Geometry check sheet. Reference: the model listing, model coordinates, mm. A direction names the side the tool comes from. Round coordinates to 2 decimals unless told otherwise and drop trailing zeros. Write each loop counter-clockwise with the first axis right and the second up, starting at its lowest first coordinate (ties: lowest second). Pieces come first, ordered by that corner, then holes. Notation, with made-up numbers: (53, 78.25) - (78, 78.25) arc R30 cw to (78, 111.25) - close; hole circle Ø7 at (17, -32.5). An arc over 180 degrees is marked (long way). Return JSON: item names as keys, results as strings.
```python
from build123d import *

# Parameters (mm, degrees)
SKETCH_W        = 20
SKETCH_H        = 40
PAD_DEPTH       = 1.75
SKETCH001_W     = 7.5
SKETCH001_H     = 5.5
PAD001_DEPTH    = 3.5
POCKET_DEPTH    = 5.5
SKETCH003_W     = 4.5
SKETCH003_H     = 0.4
POCKET001_DEPTH = 5
SKETCH004_W     = 10
SKETCH004_H     = 7.25
PAD002_DEPTH    = 5
SKETCH005_W     = 8.4
SKETCH005_H     = 4
POCKET002_DEPTH = 5
SKETCH006_W     = 0.8
SKETCH006_H     = 0.8
PAD003_DEPTH    = 4.5
SKETCH007_W     = 6
SKETCH007_H     = 6
SKETCH007_W_2   = 4.5
SKETCH007_H_2   = 4.5
SKETCH007_W_3   = 0.75
SKETCH007_H_3   = 1.5
SKETCH007_W_4   = 2.9
SKETCH007_H_4   = 1.2
SKETCH007_W_5   = 1.5
SKETCH007_H_5   = 0.75
PAD004_DEPTH    = 0.5
SKETCH008_W     = 3
SKETCH008_H     = 4
PAD005_DEPTH    = 1
SKETCH009_R     = 0.8
PAD006_DEPTH    = 0.75
SKETCH010_W     = 6
SKETCH010_H     = 5
POCKET003_DEPTH = 0.5


with BuildPart() as part:
    # Sketch → Pad (new body)
    with BuildSketch(Plane.XY):
        Rectangle(SKETCH_W, SKETCH_H)
    extrude(amount=PAD_DEPTH)

    # Sketch001 (on Face6 of Pad) → Pad001 (join)
    with BuildSketch(Plane.XY.offset(1.75)):
        with Locations((0, -17.75)):
            Rectangle(SKETCH001_W, SKETCH001_H)
    extrude(amount=PAD001_DEPTH)

    # Sketch002 (on Face11 of Pad001) → Pocket (cut)
    with BuildSketch(Plane.XZ.offset(20.5)):
        Polygon((-3.75, 5.25), (-3.75, 4.5), (-3.25, 5.25), align=None)
        Polygon((-3.75, 1.75), (-3.75, 3.5), (-2.75, 1.75), align=None)
    pocket = extrude(amount=-POCKET_DEPTH, mode=Mode.SUBTRACT)

    # Mirrored: Pocket across YZ
    add(pocket.mirror(Plane.YZ), mode=Mode.SUBTRACT)

    # Sketch003 (on Face10 of Mirrored) → Pocket001 (cut)
    with BuildSketch(Plane.XZ.offset(20.5)):
        Polygon((-3.166667, 5), (-3.5, 4.5), (-3.5, 3.75), (-2.5, 2), (2.5, 2), (3.5, 3.75), (3.5, 4.5), (3.166667, 5), align=None)
        with Locations((0, 4.1)):
            Rectangle(SKETCH003_W, SKETCH003_H, mode=Mode.SUBTRACT)
    extrude(amount=-POCKET001_DEPTH, mode=Mode.SUBTRACT)

    # Sketch004 (on Face5 of Pocket001) → Pad002 (join)
    with BuildSketch(Plane.XY.offset(1.75)):
        with Locations((0, 16.875)):
            Rectangle(SKETCH004_W, SKETCH004_H)
    extrude(amount=PAD002_DEPTH)

    # Sketch005 (on Face15 of Pad002) → Pocket002 (cut)
    with BuildSketch(Plane(origin=(0, 20.5, 0), x_dir=(-1, 0, 0), z_dir=(0, 1, 0))):
        with Locations((0, 4.25)):
            Rectangle(SKETCH005_W, SKETCH005_H)
    extrude(amount=-POCKET002_DEPTH, mode=Mode.SUBTRACT)

    # Sketch006 (on Face35 of Pocket002) → Pad003 (join)
    with BuildSketch(Plane(origin=(0, 15.5, 0), x_dir=(-1, 0, 0), z_dir=(0, 1, 0))):
        with Locations((-2.76, 4.25)):
            Rectangle(SKETCH006_W, SKETCH006_H)
        with Locations((-0.92, 4.25)):
            Rectangle(SKETCH006_W, SKETCH006_H)
        with Locations((0.92, 4.25)):
            Rectangle(SKETCH006_W, SKETCH006_H)
        with Locations((2.76, 4.25)):
            Rectangle(SKETCH006_W, SKETCH006_H)
    extrude(amount=PAD003_DEPTH)

    # Sketch007 (on Face5 of Pad003) → Pad004 (join)
    with BuildSketch(Plane.XY.offset(1.75)):
        with Locations((-3.25, -8)):
            Rectangle(SKETCH007_W, SKETCH007_H)
        with Locations((0, 3.5)):
            Rectangle(SKETCH007_W_2, SKETCH007_H_2)
        with Locations((-8.875, 8.35)):
            Rectangle(SKETCH007_W_3, SKETCH007_H_3)
        with Locations((-6.925, 8.35)):
            Rectangle(SKETCH007_W_3, SKETCH007_H_3)
        with Locations((-4.975, 8.35)):
            Rectangle(SKETCH007_W_3, SKETCH007_H_3)
        with Locations((-3.025, 8.35)):
            Rectangle(SKETCH007_W_3, SKETCH007_H_3)
        with Locations((0, 8.35)):
            Rectangle(SKETCH007_W_4, SKETCH007_H_4)
        with Locations((3.7, 9.55)):
            Rectangle(SKETCH007_W_5, SKETCH007_H_5)
        with Locations((7.15, 9.55)):
            Rectangle(SKETCH007_W_4, SKETCH007_H_4)
        with Locations((7.15, 12.03)):
            Rectangle(SKETCH007_W_3, SKETCH007_H_3)
        with Locations((7.15, 7.275)):
            Rectangle(SKETCH007_W_5, SKETCH007_H_5)
        with Locations((-5, -4.125)):
            Rectangle(SKETCH007_W_5, SKETCH007_H_5)
        with Locations((-2.5, -4.125)):
            Rectangle(SKETCH007_W_5, SKETCH007_H_5)
        with Locations((2.5, -11.375)):
            Rectangle(SKETCH007_W_5, SKETCH007_H_5)
        with Locations((-7.125, -5.75)):
            Rectangle(SKETCH007_W_3, SKETCH007_H_3)
        with Locations((-7.5, -7.375)):
            Rectangle(SKETCH007_W_5, SKETCH007_H_5)
        with Locations((1.5, -1.5)):
            Rectangle(SKETCH007_W_5, SKETCH007_H_5)
        with Locations((3.125, -1.875)):
            Rectangle(SKETCH007_W_3, SKETCH007_H_3)
    extrude(amount=PAD004_DEPTH)

    # Sketch008 (on Face5 of Pad004) → Pad005 (join)
    with BuildSketch(Plane.XY.offset(1.75)):
        with Locations((-8, -1.75)):
            Rectangle(SKETCH008_W, SKETCH008_H)
    extrude(amount=PAD005_DEPTH)

    # Sketch009 (on Face103 of Pad005) → Pad006 (join)
    with BuildSketch(Plane.XY.offset(2.75)):
        with Locations((-8, -1.75)):
            Circle(SKETCH009_R)
    extrude(amount=PAD006_DEPTH)

    # Sketch010 (on Face94 of Pad006) → Pocket003 (cut)
    with BuildSketch(Plane.XY.offset(6.75)):
        with Locations((0, 18)):
            Rectangle(SKETCH010_W, SKETCH010_H)
    extrude(amount=-POCKET003_DEPTH, mode=Mode.SUBTRACT)


solid = part.part
```
(1) Section check B-B, the plane z = 1. Enter the section's corners in (x, y).
Response values:
{"outline": "(-10, -20) - (10, -20) - (10, 20) - (-10, 20) - close"}
(2) Material ranges on line 1 along Y through (x, z) = (-1.5, 2.5); line 2 along Z through (x, y) = (2, -7); line 3 along Z through (x, y) = (1, 2), recorded low to high. Write a range as [from, to].
Response values:
{"line 1": "y = [-15.5, -15], [13.25, 15.5]", "line 2": "z = [0, 1.75]", "line 3": "z = [0, 2.25]"}
(3) Section check D-D, the plane y = 14. Enter the section's corners in (x, z), plus the area to 3 significant figures.
Response values:
{"outline": "(-10, 0) - (10, 0) - (10, 1.75) - (5, 1.75) - (5, 6.75) - (-5, 6.75) - (-5, 1.75) - (-10, 1.75) - close", "area": "85.0 mm^2"}
(4) Section check C-C, the plane y = -10. Enter the section's corners in (x, z), plus the area to 3 significant figures.
Response values:
{"outline": "(-10, 0) - (10, 0) - (10, 1.75) - (-0.25, 1.75) - (-0.25, 2.25) - (-6.25, 2.25) - (-6.25, 1.75) - (-10, 1.75) - close", "area": "38.0 mm^2"}
(5) Access from +Z, -Z, +X, -X, +Y, -Y to the whole of each face (thin tool, end or side, straight path). Record for faces 4 (the face through (3.75, -18, 4)), 5 (the face through (3.16, 17.7, 4.2)), 6 (the face through (-1.32, 17.7, 4.2)).
Response values:
{"face 4": "+Z, +X, -Y", "face 5": "+Y", "face 6": "+Z, +Y"}
(6) Release check for a two-part mould opening along Y. For faces 1 (the face through (-8.59, -1.21, 3.12)), 2 (the face through (-4.2, 18, 4)), 3 (the face through (-3, -8, 2.25)) record: pulls with the +Y half, pulls with the -Y half, needs draft (parallel to the pull), parting line crosses it, or undercut.
Response values:
{"face 1": "parting line crosses it", "face 2": "needs draft", "face 3": "undercut"}
(7) Gauge pin test, flat ends, axial feed: pin 1 (2 mm diameter, centred on x = 8, z = 5, fed in from +Y); pin 2 (0.9 mm diameter, centred on x = -2.5, z = 4, fed in from +Y). Record the tip position at first contact, or that the pin passes through.
Response values:
{"pin 1": "passes through", "pin 2": "stops at y = 20"}
(8) Section check A-A, the plane y = 8.5. Enter the section's corners in (x, z).
Response values:
{"outline": "(-10, 0) - (10, 0) - (10, 1.75) - (1.45, 1.75) - (1.45, 2.25) - (-1.45, 2.25) - (-1.45, 1.75) - (-2.65, 1.75) - (-2.65, 2.25) - (-3.4, 2.25) - (-3.4, 1.75) - (-4.6, 1.75) - (-4.6, 2.25) - (-5.35, 2.25) - (-5.35, 1.75) - (-6.55, 1.75) - (-6.55, 2.25) - (-7.3, 2.25) - (-7.3, 1.75) - (-8.5, 1.75) - (-8.5, 2.25) - (-9.25, 2.25) - (-9.25, 1.75) - (-10, 1.75) - close"}
